```python
from build123d import *

# Parameters (mm, degrees)
SKETCH1_W               = 48
SKETCH1_H               = 26
BOSS_EXTRUDE1_DEPTH     = 18
CUT_EXTRUDE1_DEPTH      = 1
CUT_EXTRUDE1_DEPTH_BACK = 49
SKETCH3_R               = 2
CUT_EXTRUDE2_DEPTH      = 1
CUT_EXTRUDE2_DEPTH_BACK = 19


with BuildPart() as part:
    # Sketch1 → Boss-Extrude1 (new body)
    with BuildSketch(Plane(origin=(0, 0, 0), x_dir=(1, 0, 0), z_dir=(0, 1, 0))):
        with Locations((24, 13)):
            Rectangle(SKETCH1_W, SKETCH1_H)
    extrude(amount=BOSS_EXTRUDE1_DEPTH)

    # Sketch2 → Cut-Extrude1 (cut, two sides)
    with BuildSketch(Plane(origin=(48, 0, 0), x_dir=(0, 0, -1), z_dir=(1, 0, 0))) as cut_extrude1_sk:
        Polygon((6, 10), (20, 10), (18.236730193, 0), (7.763269807, 0), align=None)
    extrude(amount=CUT_EXTRUDE1_DEPTH, mode=Mode.SUBTRACT)
    extrude(cut_extrude1_sk.sketch, amount=-CUT_EXTRUDE1_DEPTH_BACK, mode=Mode.SUBTRACT)

    # Sketch3 → Cut-Extrude2 (cut, two sides)
    with BuildSketch(Plane(origin=(0, 18, 0), x_dir=(1, 0, 0), z_dir=(0, 1, 0))) as cut_extrude2_sk:
        with Locations((5, 13)):
            Circle(SKETCH3_R)
    extrude(amount=CUT_EXTRUDE2_DEPTH, mode=Mode.SUBTRACT)
    extrude(cut_extrude2_sk.sketch, amount=-CUT_EXTRUDE2_DEPTH_BACK, mode=Mode.SUBTRACT)


solid = part.part
```
Could you check a few things on this model? Use its own coordinates, in mm. A direction names the side the tool comes from. Coordinates: 2 decimals unless noted, no trailing zeros. Write each loop counter-clockwise with the first axis right and the second up, starting at its lowest first coordinate (ties: lowest second). Pieces come first, ordered by that corner, then holes. Notation, with made-up numbers: (37.5, 30) -> (43.5, 30) arc R15 cw to (43.5, 35) -> close; hole circle Ø1 at (-21, -19). An arc over 180 degrees is marked (long way). Return JSON: item names as keys, results as strings.
(1) Imagine slicing it at A-A, the plane z = -13. Please give me the cut outline in (x, y), then the cut area to 3 significant figures.
Numbers:
{"outline": "(0, 10) -> (3, 10) -> (3, 18) -> (0, 18) -> close; (7, 10) -> (48, 10) -> (48, 18) -> (7, 18) -> close", "area": "352 mm2"}
(2) I need wall thicknesses on L1, parallel to X at y = 13.5, z = -13; L2, parallel to Z at x = 5, y = 13.75; L3, parallel to Y at x = 28, z = -12.75. Which ranges of each line are inside material? Lowest first, please.
Numbers:
{"L1": "x = 0 to 3, 7 to 48", "L2": "z = -26 to -15, -11 to 0", "L3": "y = 10 to 18"}
(3) Imagine slicing it at B-B, the plane x = 5. Please give me the cut outline in (y, z), then the cut area to 3 significant figures.
Numbers:
{"outline": "(0, -26) -> (18, -26) -> (18, -15) -> (10, -15) -> (10, -20) -> (0, -18.24) -> close; (0, -7.76) -> (10, -6) -> (10, -11) -> (18, -11) -> (18, 0) -> (0, 0) -> close", "area": "314 mm2"}
(4) I'm going to push flat-ended pins straight in: pin 1 (5 mm diameter, centred on y = 7, z = -11.5, fed in from -X); pin 2 (5 mm diameter, centred on y = 9, z = -19, fed in from +X); pin 3 (4 mm diameter, centred on x = 30.5, z = -12.5, fed in from -Y). Where does each tip first touch, or does it pass through?
Numbers:
{"pin 1": "passes through", "pin 2": "stops at x = 48", "pin 3": "stops at y = 10"}
(5) Imagine slicing it at D-D, the plane x = 24.5. Please give me the cut outline in (y, z).
Numbers:
{"outline": "(0, -26) -> (18, -26) -> (18, 0) -> (0, 0) -> (0, -7.76) -> (10, -6) -> (10, -20) -> (0, -18.24) -> close"}
(6) We'd pull the mould along Z, two halves only. Please class faces 1 (the flat face through (24.3, 4.9, -6.9)), 2 (the flat face through (24, 9, -26)), 3 (the flat face through (24, 9, 0)): +Z half, -Z half, draft (parallel to the pull), parting line (faces both ways), or undercut.
Numbers:
{"face 1": "undercut", "face 2": "-Z half", "face 3": "+Z half"}
(7) Imagine slicing it at C-C, the plane y = 1.5. Please give me the cut outline in (x, z).
Numbers:
{"outline": "(0, -26) -> (48, -26) -> (48, -18.5) -> (0, -18.5) -> close; (0, -7.5) -> (48, -7.5) -> (48, 0) -> (0, 0) -> close"}
(8) Which directions (+Z, -Z, +X, -X, +Y, -Y) give clear straight access to the entire face, cutting with the end or side of a thin tool? Please do faces 4 (the flat face through (24.34, 5.07, -19.13)), 5 (the flat face through (0, 11, -13)).
Numbers:
{"face 4": "+X, -X", "face 5": "+Z, -Z, -X, +Y, -Y"}
